from build123d import *

# Parameters (mm, degrees)
SKETCH1_W               = 193
SKETCH1_H               = 116.5
BOSS_EXTRUDE5_DEPTH     = 59
SHELL4_T                = -6
SKETCH6_R               = 4
SKETCH6_R_2             = 1.75
BOSS_EXTRUDE6_DEPTH     = 4
CUT_EXTRUDE1_DEPTH      = 38
CUT_EXTRUDE1_DEPTH_BACK = 34
SKETCH9_R               = 1.75
CUT_EXTRUDE2_DEPTH      = 7
FILLET2_R               = 5
SKETCH12_W              = 6
SKETCH12_H              = 6.5
BOSS_EXTRUDE7_DEPTH     = 18
SKETCH15_W              = 6
SKETCH15_H              = 7.5
BOSS_EXTRUDE8_DEPTH     = 5
SKETCH16_W              = 7.5
SKETCH16_H              = 6
SKETCH16_W_2            = 6.75
SKETCH16_W_3            = 3.5
BOSS_EXTRUDE9_DEPTH     = 7.5
SKETCH17_W              = 6
SKETCH17_H              = 31.5
BOSS_EXTRUDE10_DEPTH    = 4
SKETCH18_W              = 6
SKETCH18_H              = 1.5
BOSS_EXTRUDE11_DEPTH    = 1.5
SKETCH19_W              = 2
SKETCH19_H              = 6
BOSS_EXTRUDE12_DEPTH    = 30
SKETCH20_W              = 9
SKETCH20_H              = 2.5
BOSS_EXTRUDE13_DEPTH    = 6
SKETCH21_W              = 6
SKETCH21_H              = 7.5
CUT_EXTRUDE3_DEPTH      = 3
SKETCH22_W              = 17.5
SKETCH22_H              = 6
CUT_EXTRUDE4_DEPTH      = 2
SKETCH23_W              = 6
SKETCH23_H              = 5
CUT_EXTRUDE5_DEPTH      = 2
SKETCH24_W              = 11
SKETCH24_H              = 6
CUT_EXTRUDE6_DEPTH      = 1.5
SKETCH25_W              = 11
SKETCH25_H              = 6
CUT_EXTRUDE7_DEPTH      = 1.5
SKETCH27_W              = 17.5
SKETCH27_H              = 6
CUT_EXTRUDE8_DEPTH      = 1.5
SKETCH32_W              = 91
SKETCH32_H              = 46
BOSS_EXTRUDE15_DEPTH    = 4
SKETCH33_W              = 2
SKETCH33_H              = 87
CUT_EXTRUDE10_DEPTH     = 44
SKETCH34_W              = 8
SKETCH34_H              = 6
CUT_EXTRUDE11_DEPTH     = 1.5
SKETCH35_W              = 6
SKETCH35_H              = 30
BOSS_EXTRUDE16_DEPTH    = 11
SKETCH36_W              = 6
SKETCH36_H              = 30
BOSS_EXTRUDE17_DEPTH    = 7
SKETCH37_W              = 6
SKETCH37_H              = 31.5
BOSS_EXTRUDE18_DEPTH    = 6
SKETCH38_W              = 6
SKETCH38_H              = 31.5
BOSS_EXTRUDE19_DEPTH    = 7


with BuildPart() as part:
    # Sketch1 → Boss-Extrude5 (new body)
    with BuildSketch(Plane(origin=(0, 0, 0), x_dir=(1, 0, 0), z_dir=(0, 1, 0))):
        with Locations((10.696891192, -0.426165803)):
            Rectangle(SKETCH1_W, SKETCH1_H)
    extrude(amount=BOSS_EXTRUDE5_DEPTH)

    # Shell4
    shell4_openings = [part.faces().sort_by_distance(p)[0] for p in [
        (10.696891192, 59, 0.426165803),
    ]]
    offset(amount=SHELL4_T, openings=shell4_openings, kind=Kind.INTERSECTION)

    # Sketch6 → Boss-Extrude6 (add)
    # profile 1 of 4: a face of its own
    with BuildSketch(Plane(origin=(0, 6, 0), x_dir=(1, 0, 0), z_dir=(0, 1, 0))):
        with Locations(Location((-69.803108808, 41.823834197, 0), (0, 0, 270))):
            Circle(SKETCH6_R)
        with Locations(Location((-69.803108808, 41.823834197, 0), (0, 0, 270))):
            Circle(SKETCH6_R_2, mode=Mode.SUBTRACT)
    # profile 2 of 4: a face of its own
    with BuildSketch(Plane(origin=(0, 6, 0), x_dir=(1, 0, 0), z_dir=(0, 1, 0))):
        with Locations(Location((90.196891192, 41.823834197, 0), (0, 0, 270))):
            Circle(SKETCH6_R)
        with Locations(Location((90.196891192, 41.823834197, 0), (0, 0, 270))):
            Circle(SKETCH6_R_2, mode=Mode.SUBTRACT)
    # profile 3 of 4: a face of its own
    with BuildSketch(Plane(origin=(0, 6, 0), x_dir=(1, 0, 0), z_dir=(0, 1, 0))):
        with Locations(Location((90.196891192, -38.426165803, 0), (0, 0, 270))):
            Circle(SKETCH6_R)
        with Locations(Location((90.196891192, -38.426165803, 0), (0, 0, 270))):
            Circle(SKETCH6_R_2, mode=Mode.SUBTRACT)
    # profile 4 of 4: a face of its own
    with BuildSketch(Plane(origin=(0, 6, 0), x_dir=(1, 0, 0), z_dir=(0, 1, 0))):
        with Locations(Location((-69.803108808, -38.426165803, 0), (0, 0, 270))):
            Circle(SKETCH6_R)
        with Locations(Location((-69.803108808, -38.426165803, 0), (0, 0, 270))):
            Circle(SKETCH6_R_2, mode=Mode.SUBTRACT)
    extrude(amount=BOSS_EXTRUDE6_DEPTH)

    # Sketch8 → Cut-Extrude1 (cut, two sides: drawn at the far end of the back side and taken through both)
    with BuildSketch(Plane(origin=(0, 0, -57.823834197), x_dir=(-1, 0, 0), z_dir=(0, 0, -1)).offset(-CUT_EXTRUDE1_DEPTH_BACK)):
        Polygon((-85.946891192, 18.5), (-100.196891192, 18.5), (-100.196891192, 11), (-85.946891192, 11), (-63.946891192, 11), (-45.946891192, 11), (10.053108808, 11), (61.053108808, 11), (61.053108808, 41), (10.053108808, 41), (10.053108808, 42.5), (-45.946891192, 42.5), (-45.946891192, 25), (-63.946891192, 25), (-63.946891192, 18.5), align=None)
    extrude(amount=CUT_EXTRUDE1_DEPTH + CUT_EXTRUDE1_DEPTH_BACK, mode=Mode.SUBTRACT)

    # Sketch9 → Cut-Extrude2 (cut)
    with BuildSketch(Plane(origin=(0, 59, 0), x_dir=(1, 0, 0), z_dir=(0, 1, 0))):
        with Locations(Location((-82.803108808, 54.823834197, 0), (0, 0, 270))):
            Circle(SKETCH9_R)
        with Locations(Location((104.196891192, 54.823834197, 0), (0, 0, 270))):
            Circle(SKETCH9_R)
        with Locations(Location((-82.803108808, -55.676165803, 0), (0, 0, 270))):
            Circle(SKETCH9_R)
        with Locations(Location((104.196891192, -55.676165803, 0), (0, 0, 270))):
            Circle(SKETCH9_R)
    extrude(amount=-CUT_EXTRUDE2_DEPTH, mode=Mode.SUBTRACT)

    # Fillet2
    fillet2_edges = [part.edges().sort_by_distance(p)[0] for p in [
        (10.696891192, 0, -57.823834197),
        (107.196891192, 0, 0.426165803),
        (10.696891192, 0, 58.676165803),
        (-85.803108808, 0, 0.426165803),
    ]]
    fillet(fillet2_edges, radius=FILLET2_R)

    # Sketch12 → Boss-Extrude7 (add)
    with BuildSketch(Plane.ZY.offset(-63.946891192)):
        with Locations((-54.823834197, 21.75)):
            Rectangle(SKETCH12_W, SKETCH12_H)
    extrude(amount=BOSS_EXTRUDE7_DEPTH)

    # Sketch15 → Boss-Extrude8 (add)
    with BuildSketch(Plane.ZY.offset(-100.196891192)):
        with Locations((-54.823834197, 14.75)):
            Rectangle(SKETCH15_W, SKETCH15_H)
    extrude(amount=BOSS_EXTRUDE8_DEPTH)

    # Sketch16 → Boss-Extrude9 (add)
    with BuildSketch(Plane.XZ.offset(-18.5)):
        with Locations((83.446891192, -54.823834197)):
            Rectangle(SKETCH16_W, SKETCH16_H)
        with Locations((61.821891192, -54.823834197)):
            Rectangle(SKETCH16_W_2, SKETCH16_H)
        with Locations((47.696891192, -54.823834197)):
            Rectangle(SKETCH16_W_3, SKETCH16_H)
    extrude(amount=BOSS_EXTRUDE9_DEPTH)

    # Sketch17 → Boss-Extrude10 (add)
    with BuildSketch(Plane.ZY.offset(-45.946891192)):
        with Locations((-54.823834197, 26.75)):
            Rectangle(SKETCH17_W, SKETCH17_H)
    extrude(amount=BOSS_EXTRUDE10_DEPTH)

    # Sketch18 → Boss-Extrude11 (add)
    with BuildSketch(Plane(origin=(-10.053108808, 0, 0), x_dir=(0, 0, -1), z_dir=(1, 0, 0))):
        with Locations((54.823834197, 41.75)):
            Rectangle(SKETCH18_W, SKETCH18_H)
    extrude(amount=BOSS_EXTRUDE11_DEPTH)

    # Sketch19 → Boss-Extrude12 (add)
    with BuildSketch(Plane.XZ.offset(-41)):
        with Locations((-9.553108808, -54.823834197)):
            Rectangle(SKETCH19_W, SKETCH19_H)
    extrude(amount=BOSS_EXTRUDE12_DEPTH)

    # Sketch20 → Boss-Extrude13 (add)
    with BuildSketch(Plane(origin=(0, 0, -57.823834197), x_dir=(-1, 0, 0), z_dir=(0, 0, -1))):
        with Locations((-53.946891192, 17.25)):
            Rectangle(SKETCH20_W, SKETCH20_H)
    extrude(amount=-BOSS_EXTRUDE13_DEPTH)

    # Sketch21 → Cut-Extrude3 (cut)
    with BuildSketch(Plane.ZY.offset(-79.696891192)):
        with Locations((-54.823834197, 14.75)):
            Rectangle(SKETCH21_W, SKETCH21_H)
    extrude(amount=-CUT_EXTRUDE3_DEPTH, mode=Mode.SUBTRACT)

    # Sketch22 → Cut-Extrude4 (cut)
    with BuildSketch(Plane.XZ.offset(-18.5)):
        with Locations((73.946891192, -54.823834197)):
            Rectangle(SKETCH22_W, SKETCH22_H)
    extrude(amount=-CUT_EXTRUDE4_DEPTH, mode=Mode.SUBTRACT)

    # Sketch23 → Cut-Extrude5 (cut)
    with BuildSketch(Plane.ZY.offset(-58.446891192)):
        with Locations((-54.823834197, 13.5)):
            Rectangle(SKETCH23_W, SKETCH23_H)
    extrude(amount=-CUT_EXTRUDE5_DEPTH, mode=Mode.SUBTRACT)

    # Sketch24 → Cut-Extrude6 (cut)
    with BuildSketch(Plane.XZ.offset(-16)):
        with Locations((54.946891192, -54.823834197)):
            Rectangle(SKETCH24_W, SKETCH24_H)
    extrude(amount=-CUT_EXTRUDE6_DEPTH, mode=Mode.SUBTRACT)

    # Sketch25 → Cut-Extrude7 (cut)
    with BuildSketch(Plane(origin=(0, 11, 0), x_dir=(1, 0, 0), z_dir=(0, 1, 0))):
        with Locations((54.946891192, 54.823834197)):
            Rectangle(SKETCH25_W, SKETCH25_H)
    extrude(amount=-CUT_EXTRUDE7_DEPTH, mode=Mode.SUBTRACT)

    # Sketch27 → Cut-Extrude8 (cut)
    with BuildSketch(Plane(origin=(0, 11, 0), x_dir=(1, 0, 0), z_dir=(0, 1, 0))):
        with Locations((73.946891192, 54.823834197)):
            Rectangle(SKETCH27_W, SKETCH27_H)
    extrude(amount=-CUT_EXTRUDE8_DEPTH, mode=Mode.SUBTRACT)

    # Sketch32 → Boss-Extrude15 (add)
    with BuildSketch(Plane(origin=(107.196891192, 0, 0), x_dir=(0, 0, -1), z_dir=(1, 0, 0))):
        with Locations((-0.426165803, 36)):
            Rectangle(SKETCH32_W, SKETCH32_H)
    extrude(amount=BOSS_EXTRUDE15_DEPTH)

    # Sketch33 → Cut-Extrude10 (cut)
    with BuildSketch(Plane(origin=(0, 59, 0), x_dir=(1, 0, 0), z_dir=(0, 1, 0))):
        with Locations((108.196891192, -0.426165803)):
            Rectangle(SKETCH33_W, SKETCH33_H)
    extrude(amount=-CUT_EXTRUDE10_DEPTH, mode=Mode.SUBTRACT)

    # Sketch34 → Cut-Extrude11 (cut)
    with BuildSketch(Plane(origin=(0, 11, 0), x_dir=(1, 0, 0), z_dir=(0, 1, 0))):
        with Locations((91.196891192, 54.823834197)):
            Rectangle(SKETCH34_W, SKETCH34_H)
    extrude(amount=-CUT_EXTRUDE11_DEPTH, mode=Mode.SUBTRACT)

    # Sketch35 → Boss-Extrude16 (add)
    with BuildSketch(Plane.ZY.offset(10.553108808)):
        with Locations((-54.823834197, 26)):
            Rectangle(SKETCH35_W, SKETCH35_H)
    extrude(amount=BOSS_EXTRUDE16_DEPTH)

    # Sketch36 → Boss-Extrude17 (add)
    with BuildSketch(Plane(origin=(-61.053108808, 0, 0), x_dir=(0, 0, -1), z_dir=(1, 0, 0))):
        with Locations((54.823834197, 26)):
            Rectangle(SKETCH36_W, SKETCH36_H)
    extrude(amount=BOSS_EXTRUDE17_DEPTH)

    # Sketch37 → Boss-Extrude18 (add)
    with BuildSketch(Plane(origin=(-8.553108808, 0, 0), x_dir=(0, 0, -1), z_dir=(1, 0, 0))):
        with Locations((54.823834197, 26.75)):
            Rectangle(SKETCH37_W, SKETCH37_H)
    extrude(amount=BOSS_EXTRUDE18_DEPTH)

    # Sketch38 → Boss-Extrude19 (add)
    with BuildSketch(Plane.ZY.offset(-41.946891192)):
        with Locations((-54.823834197, 26.75)):
            Rectangle(SKETCH38_W, SKETCH38_H)
    extrude(amount=BOSS_EXTRUDE19_DEPTH)


solid = part.part
Here's how the part is built. I have some questions about the finished solid (model axes, mm). A direction names the side the tool comes from. Round coordinates to 2 decimals unless told otherwise and drop trailing zeros. Loops run counter-clockwise (first coordinate to the right, second up) from the corner with the lowest first, then second, coordinate; pieces in that order, holes last. Notation, with made-up numbers: (-1, -28) - (32, -28) arc R16 ccw to (32, -3) - close; hole circle Ø9 at (38.25, -17.75). An arc over 180 degrees is marked (long way). One line per question, with ' | ' between items. Start each with the question number.
Q1. I want a section at C-C (z = -23). Write out the boundary of the cut face in (x, y).
Q2. Please list where these lines run through material, in increasing order: line 1 (X direction, y = 35, z = 30); line 2 (Z direction, x = -60, y = 50); line 3 (X direction, y = 14, z = -36). Write a range as [from, to].
Q3. I want a section at A-A (x = 16.5). Write out the boundary of the cut face in (y, z).
Q4. I want a section at B-B (y = 45.5). Write out the boundary of the cut face in (x, z).
Q5. Will these pins go through, and if not, where does the flat tip stop? pin 1 (9 mm diameter, centred on x = 89.5, z = 39, fed in from +Y); pin 2 (1.8 mm diameter, centred on y = 12.5, z = -55.5, fed in from +X); pin 3 (1 mm diameter, centred on x = -82, z = 55, fed in from +Y).
Q6. I want a section at D-D (x = 55). Write out the boundary of the cut face in (y, z), then the cut area to 3 significant figures.
Q7. For faces 5 (the flat face through (49.447, 14, -55)), 6 (the flat face through (109, 36, 45.926)), 7 (the flat face through (109, 36, -45.074)), 8 (the flat face through (12, 44, -57.824)), 9 (the flat face through (-79.803, 32, 1)), which set-ups out of +Z, -Z, +X, -X, +Y, -Y let a thin tool reach every point of the face, with its end or its side?
Q8. We'd pull the mould along Z, two halves only. Please class faces 1 (the cylindrical face through (-65.837, 7.972, -42.345)), 2 (the flat face through (12, 44, -51.824)), 3 (the flat face through (95.197, 14, -55)), 4 (the cylindrical face through (12.048, 1.504, 57.25)): +Z half, -Z half, draft (parallel to the pull), parting line (faces both ways), or undercut.
Response values:
1) outline: (-85.8, 5) arc R5 ccw to (-80.8, 0) - (102.2, 0) arc R5 ccw to (107.2, 5) - (107.2, 13) - (111.2, 13) - (111.2, 59) - (109.2, 59) - (109.2, 15) - (107.2, 15) - (107.2, 59) - (101.2, 59) - (101.2, 6) - (-79.8, 6) - (-79.8, 59) - (-85.8, 59) - close
2) line 1: x = [-85.8, -79.8], [101.2, 107.2], [109.2, 111.2] | line 2: z = [-57.82, -51.82], [52.68, 58.68] | line 3: x = [-85.8, -79.8], [101.2, 111.2]
3) outline: (0, -52.82) arc R5 ccw to (5, -57.82) - (11, -57.82) - (11, -51.82) - (6, -51.82) - (6, 52.68) - (59, 52.68) - (59, 58.68) - (5, 58.68) arc R5 ccw to (0, 53.68) - close; (42.5, -57.82) - (59, -57.82) - (59, -51.82) - (42.5, -51.82) - close
4) outline: (-85.8, -57.82) - (107.2, -57.82) - (107.2, -45.07) - (111.2, -45.07) - (111.2, 45.93) - (107.2, 45.93) - (107.2, 58.68) - (-85.8, 58.68) - close; hole (-79.8, -51.82) - (101.2, -51.82) - (101.2, 52.68) - (-79.8, 52.68) - close; hole (107.2, -43.07) - (109.2, -43.07) - (109.2, 43.93) - (107.2, 43.93) - close
5) pin 1: stops at y = 10 | pin 2: stops at x = 107.2 | pin 3: stops at y = 52
6) outline: (0, -52.82) arc R5 ccw to (5, -57.82) - (9.5, -57.82) - (9.5, -51.82) - (6, -51.82) - (6, 52.68) - (59, 52.68) - (59, 58.68) - (5, 58.68) arc R5 ccw to (0, 53.68) - close; (17.5, -57.82) - (59, -57.82) - (59, -51.82) - (17.5, -51.82) - close | area: 1,280 mm²
7) face 5: -Z | face 6: +Z, +X, +Y, -Y | face 7: -Z, +X, +Y, -Y | face 8: -Z, +X, -X, +Y, -Y | face 9: +Y
8) face 1: undercut | face 2: undercut | face 3: draft | face 4: +Z half
